from build123d import *

# Parameters (mm, degrees)
BOSS_EXTRUDE2_DEPTH     = 32
CUT_EXTRUDE1_DEPTH      = 10
CUT_EXTRUDE1_DEPTH_BACK = 40
SKETCH2_R               = 25
CUT_EXTRUDE2_START      = -2
SKETCH3_R               = 39.875
CUT_EXTRUDE2_DEPTH      = 40
FILLET1_R               = 8
FILLET2_R               = 2
CUT_EXTRUDE3_DEPTH      = 10
CUT_EXTRUDE3_DEPTH_BACK = 10
SKETCH5_R               = 1.7
CUT_EXTRUDE4_DEPTH      = 5
CUT_EXTRUDE4_DEPTH_BACK = 7
SKETCH6_R               = 1.5


with BuildPart() as part:
    # Sketch4 → Boss-Extrude2 (new body)
    with BuildSketch(Plane(origin=(0, 0, 0), x_dir=(0, 0, -1), z_dir=(1, 0, 0))):
        with BuildLine():
            Line((-60.875, -40.875), (-60.875, -45))
            Line((-60.875, -45), (60.875, -45))
            Line((60.875, -45), (60.875, -40.875))
            Line((60.875, -40.875), (40.875, -40.875))
            Line((40.875, -40.875), (40.875, 0))
            ThreePointArc((40.875, 0), (0, 40.875), (-40.875, 0))
            Line((-40.875, 0), (-40.875, -40.875))
            Line((-40.875, -40.875), (-60.875, -40.875))
        make_face()
    extrude(amount=-BOSS_EXTRUDE2_DEPTH)

    # Sketch2 → Cut-Extrude1 (cut, two sides: drawn at the far end of the back side and taken through both)
    with BuildSketch(Plane(origin=(0, 0, 0), x_dir=(0, 0, -1), z_dir=(1, 0, 0)).offset(-CUT_EXTRUDE1_DEPTH_BACK)):
        with Locations(Location((0, 0, 0), (0, 0, 180))):
            Circle(SKETCH2_R)
    extrude(amount=CUT_EXTRUDE1_DEPTH + CUT_EXTRUDE1_DEPTH_BACK, mode=Mode.SUBTRACT)

    # Sketch3 → Cut-Extrude2 (cut)
    with BuildSketch(Plane(origin=(0, 0, 0), x_dir=(0, 0, -1), z_dir=(1, 0, 0)).offset(CUT_EXTRUDE2_START)):
        Circle(SKETCH3_R)
    extrude(amount=-CUT_EXTRUDE2_DEPTH, mode=Mode.SUBTRACT)

    # Fillet1
    fillet1_edges = [part.edges().sort_by_distance(p)[0] for p in [
        (-16, -40.875, -40.875),
        (-16, -40.875, 40.875),
    ]]
    fillet(fillet1_edges, radius=FILLET1_R)

    # Fillet2
    fillet2_edges = [part.edges().sort_by_distance(p)[0] for p in [
        (-16, -40.875, -60.875),
        (-16, -40.875, 60.875),
    ]]
    fillet(fillet2_edges, radius=FILLET2_R)

    # Sketch5 → Cut-Extrude3 (cut, two sides: drawn at the far end of the back side and taken through both)
    with BuildSketch(Plane(origin=(0, 0, 0), x_dir=(0, 0, -1), z_dir=(1, 0, 0)).offset(-CUT_EXTRUDE3_DEPTH_BACK)):
        with Locations(Location((36.5, 0, 0), (0, 0, 180))):
            Circle(SKETCH5_R)
        with Locations(Location((27.960622174, -23.461747754, 0), (0, 0, 180))):
            Circle(SKETCH5_R)
        with Locations(Location((6.338158485, -35.945482985, 0), (0, 0, 180))):
            Circle(SKETCH5_R)
        with Locations(Location((-18.25, -31.609927238, 0), (0, 0, 180))):
            Circle(SKETCH5_R)
        with Locations(Location((-34.298780659, -12.483735231, 0), (0, 0, 180))):
            Circle(SKETCH5_R)
        with Locations(Location((-34.298780659, 12.483735231, 0), (0, 0, 180))):
            Circle(SKETCH5_R)
        with Locations(Location((-18.25, 31.609927238, 0), (0, 0, 180))):
            Circle(SKETCH5_R)
        with Locations(Location((6.338158485, 35.945482985, 0), (0, 0, 180))):
            Circle(SKETCH5_R)
        with Locations(Location((27.960622174, 23.461747754, 0), (0, 0, 180))):
            Circle(SKETCH5_R)
        with Locations(Location((34.298780659, -12.483735231, 0), (0, 0, 180))):
            Circle(SKETCH5_R)
        with Locations(Location((-27.960622174, -23.461747754, 0), (0, 0, 180))):
            Circle(SKETCH5_R)
        with Locations(Location((-6.338158485, 35.945482985, 0), (0, 0, 180))):
            Circle(SKETCH5_R)
    extrude(amount=CUT_EXTRUDE3_DEPTH + CUT_EXTRUDE3_DEPTH_BACK, mode=Mode.SUBTRACT)

    # Sketch6 → Cut-Extrude4 (cut, two sides: drawn at the far end of the back side and taken through both)
    with BuildSketch(Plane(origin=(0, -45, 0), x_dir=(-1, 0, 0), z_dir=(0, -1, 0)).offset(-CUT_EXTRUDE4_DEPTH_BACK)):
        with Locations(Location((7.5, 50.875, 0), (0, 0, 270))):
            Circle(SKETCH6_R)
        with Locations(Location((24.5, 50.875, 0), (0, 0, 270))):
            Circle(SKETCH6_R)
        with Locations(Location((24.5, -50.875, 0), (0, 0, 270))):
            Circle(SKETCH6_R)
        with Locations(Location((7.5, -50.875, 0), (0, 0, 270))):
            Circle(SKETCH6_R)
    extrude(amount=CUT_EXTRUDE4_DEPTH + CUT_EXTRUDE4_DEPTH_BACK, mode=Mode.SUBTRACT)


solid = part.part
Check sheet for the modelled part. Datum: model origin and axes. Units: mm. A direction names the side the tool comes from. Round coordinates to 2 decimals unless told otherwise and drop trailing zeros. Write each loop counter-clockwise with the first axis right and the second up, starting at its lowest first coordinate (ties: lowest second). Pieces come first, ordered by that corner, then holes. Notation, with made-up numbers: (-13, 74.5) - (20, 74.5) arc R27 cw to (20, 105.5) - close; hole circle Ø5 at (42, 87.25). An arc over 180 degrees is marked (long way). Return JSON: item names as keys, results as strings.
Q1. Cross-section at C-C (x = -18.5). Record the boundary of the cut face in (y, z) (3 decimals).
Returned:
{"outline": "(-45, -60.875) - (-42.875, -60.875) arc R2 ccw to (-40.875, -58.875) - (-40.875, -48.875) arc R8 cw to (-32.875, -40.875) - (0, -40.875) arc R40.875 ccw to (0, 40.875) - (-32.875, 40.875) arc R8 cw to (-40.875, 48.875) - (-40.875, 58.875) arc R2 ccw to (-42.875, 60.875) - (-45, 60.875) - close; hole circle Ø79.75 at (0, 0)"}
Q2. Draft check along X on faces 4 (the flat face through (-32, -40.03, 0.28)), 5 (the cylindrical face through (-16.224, -38.594, -43.281)), 6 (the cylindrical face through (-25.514, -42.909, 49.769)). Enter one of: released by +X, released by -X, zero draft, split by the parting line, or undercut.
Returned:
{"face 4": "released by -X", "face 5": "zero draft", "face 6": "undercut"}
Q3. Depth check by flat-ended pin: P1, Ø2, axis at y = -12.48, z = 34.3, coming from the +X side; P2, Ø11, axis at x = -23.5, z = 54, coming from the +Y side; P3, Ø4, axis at x = -27.5, y = -28.5, coming from the +Z side (3 decimals); P4, Ø2, axis at x = -18.5, z = -38.5, coming from the +Y side. Enter the tip coordinate at first touch or a pass-through.
Returned:
{"P1": "passes through", "P2": "stops at y = -40.87", "P3": "stops at z = 40.875", "P4": "stops at y = 16.26"}
Q4. Cross-section at B-B (z = 0). Record the boundary of the cut face in (x, y) (3 decimals).
Returned:
{"outline": "(-32, -45) - (0, -45) - (0, -25) - (-2, -25) - (-2, -39.875) - (-32, -39.875) - close; (-32, 39.875) - (-2, 39.875) - (-2, 25) - (0, 25) - (0, 40.875) - (-32, 40.875) - close"}
Q5. Cross-section at A-A (x = -7.5). Record the boundary of the cut face in (y, z) (3 decimals), then the cut area to 3 significant figures.
Returned:
{"outline": "(-45, -60.875) - (-42.875, -60.875) arc R2 ccw to (-40.875, -58.875) - (-40.875, -52.375) - (-45, -52.375) - close; (-45, -49.375) - (-40.875, -49.375) - (-40.875, -48.875) arc R8 cw to (-32.875, -40.875) - (0, -40.875) arc R40.875 ccw to (0, 40.875) - (-32.875, 40.875) arc R8 cw to (-40.875, 48.875) - (-40.875, 49.375) - (-45, 49.375) - close; (-45, 52.375) - (-40.875, 52.375) - (-40.875, 58.875) arc R2 ccw to (-42.875, 60.875) - (-45, 60.875) - close; hole circle Ø79.75 at (0, 0)", "area": "1,470 mm²"}
Q6. Scan lines: L1, parallel to Y at x = -21, z = 0 (3 decimals); L2, parallel to Y at x = -0.65, z = 18.25; L3, parallel to Z at x = -18.5, y = -23 (3 decimals). Record each from-to range of solid material in increasing order. Write a range as from..to.
Returned:
{"L1": "y = -45..-39.875, 39.875..40.875", "L2": "y = -45..-33.31, -29.91..-17.09, 17.09..29.91, 33.31..36.57", "L3": "z = -40.875..-32.573, 32.573..40.875"}
Q7. Access from +Z, -Z, +X, -X, +Y, -Y to the whole of each face (thin tool, end or side, straight path). Record for faces 1 (the flat face through (-16, -40.875, 54)), 2 (the flat face through (-16, -40.875, -54)), 3 (the cylindrical face through (-16.79, -24.263, 31.643)).
Returned:
{"face 1": "+Z, +X, -X, +Y", "face 2": "-Z, +X, -X, +Y", "face 3": "-X"}
Q8. Cross-section at D-D (y = -5). Record the boundary of the cut face in (x, z) (3 decimals).
Returned:
{"outline": "(-32, -40.875) - (0, -40.875) - (0, -24.495) - (-2, -24.495) - (-2, -39.56) - (-32, -39.56) - close; (-32, 39.56) - (-2, 39.56) - (-2, 24.495) - (0, 24.495) - (0, 40.875) - (-32, 40.875) - close"}
